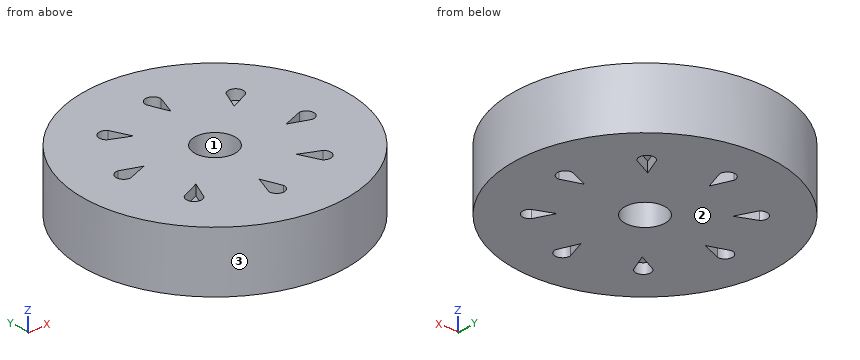
```python
from build123d import *

# Parameters (mm, degrees)
F0_R     = 20.6375
F1_DEPTH = 4.7625
F2_R     = 3.175
F4_DEPTH = 12.7
F5_DEPTH = 1.5875
F7_DEPTH = 1.5875


with BuildPart() as f1:
    # F0 (on Top) → F1 (new body, symmetric)
    with BuildSketch(Plane.XY):
        Circle(F0_R)
    extrude(amount=F1_DEPTH, both=True)

    # F2 (on Top) → F4 (cut, symmetric)
    with BuildSketch(Plane.XY):
        Circle(F2_R)
    extrude(amount=F4_DEPTH, both=True, mode=Mode.SUBTRACT)

    # F3 (on face) → F5 (cut)
    with BuildSketch(Plane.XY.offset(4.7625)):
        with BuildLine():
            Line((-5.724748, 8.25276), (-7.050308, 11.314797))
            ThreePointArc((-7.050308, 11.314797), (-8.78422, 11.409519), (-8.743804, 9.673492))
            Line((-8.743804, 9.673492), (-5.724748, 8.25276))
        make_face()
        with BuildLine():
            Line((-9.883591, 1.787574), (-12.98609, 3.015449))
            ThreePointArc((-12.98609, 3.015449), (-14.27913, 1.856367), (-13.022995, 0.657388))
            Line((-13.022995, 0.657388), (-9.883591, 1.787574))
        make_face()
        with BuildLine():
            Line((-8.25276, -5.724748), (-11.314797, -7.050308))
            ThreePointArc((-11.314797, -7.050308), (-11.409519, -8.78422), (-9.673492, -8.743804))
            Line((-9.673492, -8.743804), (-8.25276, -5.724748))
        make_face()
        with BuildLine():
            Line((-1.787574, -9.883591), (-3.015449, -12.98609))
            ThreePointArc((-3.015449, -12.98609), (-1.856367, -14.27913), (-0.657388, -13.022995))
            Line((-0.657388, -13.022995), (-1.787574, -9.883591))
        make_face()
        with BuildLine():
            Line((5.724748, -8.25276), (7.050308, -11.314797))
            ThreePointArc((7.050308, -11.314797), (8.78422, -11.409519), (8.743804, -9.673492))
            Line((8.743804, -9.673492), (5.724748, -8.25276))
        make_face()
        with BuildLine():
            Line((9.883591, -1.787574), (12.98609, -3.015449))
            ThreePointArc((12.98609, -3.015449), (14.27913, -1.856367), (13.022995, -0.657388))
            Line((13.022995, -0.657388), (9.883591, -1.787574))
        make_face()
        with BuildLine():
            Line((8.25276, 5.724748), (11.314797, 7.050308))
            ThreePointArc((11.314797, 7.050308), (11.409519, 8.78422), (9.673492, 8.743804))
            Line((9.673492, 8.743804), (8.25276, 5.724748))
        make_face()
        with BuildLine():
            Line((1.787574, 9.883591), (3.015449, 12.98609))
            ThreePointArc((3.015449, 12.98609), (1.856367, 14.27913), (0.657388, 13.022995))
            Line((0.657388, 13.022995), (1.787574, 9.883591))
        make_face()
    extrude(amount=-F5_DEPTH, mode=Mode.SUBTRACT)

    # F6 (on face) → F7 (cut)
    with BuildSketch(Plane(origin=(0, 0, -4.7625), x_dir=(1, 0, 0), z_dir=(0, 0, -1))):
        with BuildLine():
            Line((-6.830625, 8.059029), (-8.156184, 11.121066))
            ThreePointArc((-8.156184, 11.121066), (-9.890096, 11.215789), (-9.849681, 9.479761))
            Line((-9.849681, 9.479761), (-6.830625, 8.059029))
        make_face()
        with BuildLine():
            Line((-10.528575, 0.868613), (-13.631074, 2.096489))
            ThreePointArc((-13.631074, 2.096489), (-14.924114, 0.937406), (-13.66798, -0.261572))
            Line((-13.66798, -0.261572), (-10.528575, 0.868613))
        make_face()
        with BuildLine():
            Line((-8.059029, -6.830625), (-11.121066, -8.156184))
            ThreePointArc((-11.121066, -8.156184), (-11.215789, -9.890096), (-9.479761, -9.849681))
            Line((-9.479761, -9.849681), (-8.059029, -6.830625))
        make_face()
        with BuildLine():
            Line((-0.868613, -10.528575), (-2.096489, -13.631074))
            ThreePointArc((-2.096489, -13.631074), (-0.937406, -14.924114), (0.261572, -13.66798))
            Line((0.261572, -13.66798), (-0.868613, -10.528575))
        make_face()
        with BuildLine():
            Line((6.830625, -8.059029), (8.156184, -11.121066))
            ThreePointArc((8.156184, -11.121066), (9.890096, -11.215789), (9.849681, -9.479761))
            Line((9.849681, -9.479761), (6.830625, -8.059029))
        make_face()
        with BuildLine():
            Line((10.528575, -0.868613), (13.631074, -2.096489))
            ThreePointArc((13.631074, -2.096489), (14.924114, -0.937406), (13.66798, 0.261572))
            Line((13.66798, 0.261572), (10.528575, -0.868613))
        make_face()
        with BuildLine():
            Line((8.059029, 6.830625), (11.121066, 8.156184))
            ThreePointArc((11.121066, 8.156184), (11.215789, 9.890096), (9.479761, 9.849681))
            Line((9.479761, 9.849681), (8.059029, 6.830625))
        make_face()
        with BuildLine():
            Line((0.868613, 10.528575), (2.096489, 13.631074))
            ThreePointArc((2.096489, 13.631074), (0.937406, 14.924114), (-0.261572, 13.66798))
            Line((-0.261572, 13.66798), (0.868613, 10.528575))
        make_face()
    extrude(amount=-F7_DEPTH, mode=Mode.SUBTRACT)


solid = f1.part
```
Work out the finished part from the listing and answer in its coordinate system (mm). Face numbers are marked on the shaded views. Give positions to 0.01 mm unless a question says otherwise; leave off trailing zeros. Loops run counter-clockwise (first coordinate to the right, second up) from the corner with the lowest first, then second, coordinate; pieces in that order, holes last. Notation, with made-up numbers: (39.25, -9.5) - (73.25, -9.5) arc R20 cw to (73.25, 1.5) - close; hole circle Ø5 at (61, -36). An arc over 180 degrees is marked (long way). Use CSV: the item, a comma, the result in double quotes. Start each with the question number.
(1) Find section C-C, the plane x = 5. Determine the outline of the cut face in (y, z).
(2) Determine the mould class of the marked faces 1, 2 and 3 for opening direction Y: released by +Y, released by -Y, zero draft, split by the parting line, or undercut.
(3) Find section A-A, the plane z = 3.75. Count the separate pieces of the cut face and the enclosed holes in it, plus the area to 3 significant figures.
(4) Find section D-D, the plane x = -4. Determine the outline of the cut face in (y, z), plus the area to 3 significant figures.
(5) Each of these flat-tipped pins is pushed along its axis until it touches: pin 1 (0.7 mm diameter, centred on x = -1.5, y = -12.5, fed in from +Z) (3 decimals); pin 2 (0.7 mm diameter, centred on x = 1, y = -13, fed in from -Z) (3 decimals); pin 3 (4 mm diameter, centred on x = -12, z = 1.5, fed in from -Y); pin 4 (5 mm diameter, centred on x = 0, y = 0, fed in from -Z). Where does it stop, or does it pass through?
(6) Find the intervals of material crossed by L1, parallel to Y at x = 0, z = 2.25 (1 decimal); L2, parallel to Z at x = -14, y = 2 (1 decimal); L3, parallel to Y at x = -1, z = -0.75, in increasing order.
Results found:
1,outline,"(-20.02, -4.76) - (20.02, -4.76) - (20.02, 4.76) - (-20.02, 4.76) - close"
2,face 1,"undercut"
2,face 2,"zero draft"
2,face 3,"split by the parting line"
3,separate pieces,"1"
3,enclosed holes,"9"
3,area,"1,260 mm^2"
4,outline,"(-20.25, -4.76) - (20.25, -4.76) - (20.25, 4.76) - (-20.25, 4.76) - close"
4,area,"386 mm^2"
5,pin 1,"z = 3.175"
5,pin 2,"z = -3.175"
5,pin 3,"y = -18.05"
5,pin 4,"through"
6,L1,"-20.6 to -3.2, 3.2 to 20.6"
6,L2,"-4.8 to 3.2"
6,L3,"-20.61 to -3.01, 3.01 to 20.61"
